Part model, mm, in its own coordinate system. A direction names the side the tool comes from. Give positions to 0.01 mm unless a question says otherwise; leave off trailing zeros. Order: outer loops, then holes, each group sorted by start corner. A loop starts at its lowest first (then second) coordinate and runs counter-clockwise, first axis right, second up. Notation, with made-up numbers: (35, -6) - (80, -6) arc R14 ccw to (80, 13) - close; hole circle Ø7 at (-17, -25.75). An arc over 180 degrees is marked (long way). One line per item, written item: value.
Autodesk Inventor part; units mm, degrees
ref_plane "YZ Plane" through (0, 0, 0) normal (1, 0, 0) x (0, 1, 0)
ref_plane "XZ Plane" through (0, 0, 0) normal (0, 1, 0) x (-1, 0, 0)
ref_plane "XY Plane" through (0, 0, 0) normal (0, 0, 1) x (1, 0, 0)
sketch "Sketch1" plane through (0, 0, 0) normal (0, 1, 0) x (-1, 0, 0)
  line L0 (0, 165.1) -> (304.8, 76.2)
  line L1 (304.8, 76.2) -> (304.8, -76.2)
  line L2 (304.8, -76.2) -> (0, -165.1)
  line L3 (0, -165.1) -> (0, 165.1)
  point P0 (0, 0)
  point P1 (304.8, 0)
  point P2 (0, 0)
  dimension "d0" = 330.2
  dimension "d1" = 152.4
  dimension "d2" = 304.8
extrude "Extrusion1" add sketch "Sketch1" along normal blind 127
shell "Shell1" thickness 6.35 removed faces 2 at (0, 42.3333, 55.0333) at (-304.8, 42.3333, -25.4)
properties part number "feeder block" material "Aluminum 6061"
1) Slice it at B-B on z = 40. Write the cut outline in (x, y).
Answer:
outline: (-304.8, 0) - (0, 0) - (0, 6.35) - (-304.8, 6.35) - close; (-304.8, 120.65) - (0, 120.65) - (0, 127) - (-304.8, 127) - close
2) Wall check: line 1 along Y through (x, z) = (-241.5, 81.5); line 2 along Z through (x, y) = (-174.5, 26); line 3 along Z through (x, y) = (-95, 16). Give the ranges that are in metal, low to high. Write a range as [from, to].
Answer:
line 1: y = [0, 6.35], [120.65, 127]
line 2: z = [-114.2, -107.59], [107.59, 114.2]
line 3: z = [-137.39, -130.78], [130.78, 137.39]
3) Drop flat-ended pins along their axis: P1, Ø2, axis at x = -213, y = 71, coming from the +Z side; P2, Ø10, axis at x = -226, y = 100, coming from the -Z side. Give the stop position or say it passes through.
Answer:
P1: stops at z = 103.27
P2: stops at z = -100.64
4) Slice it at C-C on x = -18.5. Write the cut outline in (y, z).
Answer:
outline: (0, -159.7) - (127, -159.7) - (127, 159.7) - (0, 159.7) - close; hole (6.35, -153.09) - (120.65, -153.09) - (120.65, 153.09) - (6.35, 153.09) - close
5) Slice it at D-D on z = -142.5. Write the cut outline in (x, y), then the cut area to 3 significant figures.
Answer:
outline: (-77.49, 0) - (0, 0) - (0, 6.35) - (-54.81, 6.35) - (-54.81, 120.65) - (0, 120.65) - (0, 127) - (-77.49, 127) - close
area: 3,580 mm2
6) Two-plate mould, pull along Z, no slides. Class faces 1 (the face through (-304.8, 124, 6)), 2 (the face through (-154.53, 62.61, -120.03)), 3 (the face through (-116, 6.35, 2)): pulls with the +Z half, pulls with the -Z half, needs draft (parallel to the pull), parting line crosses it, or undercut.
Answer:
face 1: needs draft
face 2: pulls with the -Z half
face 3: undercut
7) Which spindle directions (+Z, -Z, +X, -X, +Y, -Y) get a long thin tool onto all of the face, cutting with end or side? Do faces 4 (the face through (-116, 120.65, 2)), 5 (the face through (-116, 127, 2)). Say none if no direction does.
Answer:
face 4: +X
face 5: +Z, -Z, +X, -X, +Y
8) Slice it at A-A on y = 73.5. Write the cut outline in (x, z), then the cut area to 3 significant figures.
Answer:
outline: (-304.8, -76.2) - (0, -165.1) - (0, -158.49) - (-304.8, -69.59) - close; (-304.8, 69.59) - (0, 158.49) - (0, 165.1) - (-304.8, 76.2) - close
area: 4,030 mm2
